Verification items for the finished model (mm, model axes). Face numbers are marked on the shaded views. A direction names the side the tool comes from. Coordinates: 2 decimals unless noted, no trailing zeros. Write each loop counter-clockwise with the first axis right and the second up, starting at its lowest first coordinate (ties: lowest second). Pieces come first, ordered by that corner, then holes. Notation, with made-up numbers: (71.5, 81) -> (124.5, 81) arc R24 ccw to (124.5, 93) -> close; hole circle Ø11 at (26.25, 54.5). An arc over 180 degrees is marked (long way). Use CSV: the item, a comma, the result in double quotes.
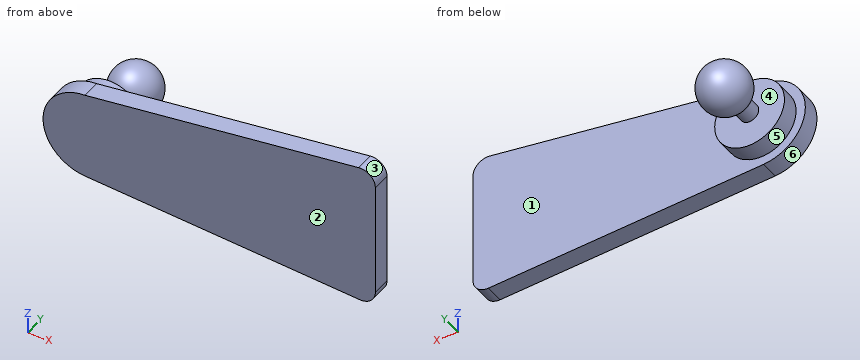
```python
from build123d import *

# Parameters (mm, degrees)
BOSS_EXTRUDE1_DEPTH = 3.175
FILLET1_R           = 2.54
SKETCH2_R           = 6.0325
BOSS_EXTRUDE3_DEPTH = 3.175
SKETCH3_R           = 1.5875
BOSS_EXTRUDE4_DEPTH = 3.175


with BuildPart() as part:
    # Sketch1 → Boss-Extrude1 (new body)
    with BuildSketch(Plane(origin=(0, 0, 0), x_dir=(1, 0, 0), z_dir=(0, 1, 0))):
        with BuildLine():
            Line((15.837639572, 15.574796876), (15.837639572, -9.825203124))
            Line((15.837639572, -9.825203124), (-34.402531646, -2.304219409))
            ThreePointArc((-34.402531646, -2.304219409), (-41.632773479, 5.315780591), (-34.402531646, 12.935780591))
            Line((-34.402531646, 12.935780591), (15.837639572, 15.574796876))
        make_face()
    extrude(amount=BOSS_EXTRUDE1_DEPTH)

    # Fillet1
    fillet1_edges = [part.edges().sort_by_distance(p)[0] for p in [
        (15.837639572, 1.5875, -15.574796876),
        (15.837639572, 1.5875, 9.825203124),
    ]]
    fillet(fillet1_edges, radius=FILLET1_R)

    # Sketch2 → Boss-Extrude3 (add)
    with BuildSketch(Plane(origin=(0, 3.175, 0), x_dir=(1, 0, 0), z_dir=(0, 1, 0))):
        with Locations(Location((-34.002268199, 5.315780591, 0), (0, 0, 270))):
            Circle(SKETCH2_R)
    extrude(amount=BOSS_EXTRUDE3_DEPTH)

    # Sketch3 → Boss-Extrude4 (add)
    with BuildSketch(Plane(origin=(0, 6.35, 0), x_dir=(1, 0, 0), z_dir=(0, 1, 0))):
        with Locations(Location((-34.002268199, 5.315780591, 0), (0, 0, 270))):
            Circle(SKETCH3_R)
    extrude(amount=BOSS_EXTRUDE4_DEPTH)

    # Sketch6 → Revolve1 (revolve)
    with BuildSketch(Plane.XY.offset(-5.315780591)):
        with BuildLine():
            Line((-34.008296726, 17.526), (-34.008296726, 8.89))
            ThreePointArc((-34.008296726, 8.89), (-38.326296726, 13.208), (-34.008296726, 17.526))
        make_face()
    revolve(axis=Axis((-34.008296726, 17.526, -5.315780591), (0, -1, 0)))


solid = part.part
```
1) Gauge pin test, flat ends, axial feed: pin 1 (5 mm diameter, centred on x = -33.5, z = -9.5, fed in from -Y); pin 2 (10 mm diameter, centred on y = 3, z = 6, fed in from -X); pin 3 (6 mm diameter, centred on y = 8.5, z = -3, fed in from -X). Record the tip position at first contact, or that the pin passes through.
Return value:
pin 1,"y = 0"
pin 2,"x = -38.28"
pin 3,"x = -40.03"
2) Cross-section at B-B (x = -37). Record the boundary of the cut face in (y, z) (3 decimals), plus the area to 3 significant figures.
Return value:
outline,"(0, -12.333) -> (3.175, -12.333) -> (3.175, -10.551) -> (6.35, -10.551) -> (6.35, -0.081) -> (3.175, -0.081) -> (3.175, 1.701) -> (0, 1.701) -> close; circle Ø6.227 at (13.208, -5.316)"
area,"108 mm2"
3) Set-up check for the marked faces 5 and 6: record each of +Z, -Z, +X, -X, +Y, -Y from which the full face is reachable in a straight line by a thin tool's end or side.
Return value:
face 5,"+Y"
face 6,"-X, +Y, -Y"
4) Cross-section at C-C (z = -0.25). Record the boundary of the cut face in (x, y) (3 decimals).
Return value:
outline,"(-39.709, 0) -> (15.838, 0) -> (15.838, 3.175) -> (-30.727, 3.175) -> (-30.727, 6.35) -> (-37.278, 6.35) -> (-37.278, 3.175) -> (-39.709, 3.175) -> close"
5) Cross-section at D-D (y = 11.25). Record the boundary of the cut face in (x, z).
Return value:
outline,"circle Ø7.7 at (-34.01, -5.32)"
6) Mould release check, pull along Y, two halves, no side actions. Record for the marked faces 1, 2, 3 and 4: released by +Y, released by -Y, zero draft, split by the parting line, or undercut.
Return value:
face 1,"released by +Y"
face 2,"released by -Y"
face 3,"zero draft"
face 4,"undercut"
7) Scan lines: L1, parallel to Y at x = 8.5, z = 2.75 (3 decimals); L2, parallel to X at y = 15.5, z = -7.5; L3, parallel to Z at x = -14, y = 1.5. Record each from-to range of solid material in increasing order.
Return value:
L1,"0 to 3.175"
L2,"-36.94 to -31.07"
L3,"-14.01 to 5.36"
